Autodesk Inventor part; units mm, degrees
ref_plane "YZ Plane" through (0, 0, 0) normal (1, 0, 0) x (0, 1, 0)
ref_plane "XZ Plane" through (0, 0, 0) normal (0, 1, 0) x (-1, 0, 0)
ref_plane "XY Plane" through (0, 0, 0) normal (0, 0, 1) x (1, 0, 0)
sketch "Sketch1" plane through (0, 0, 0) normal (0, 0, 1) x (1, 0, 0)
  line L0 (-17.5524, 1.6365) -> (20.5476, 1.6365)
  line L1 (20.5476, 1.6365) -> (20.5476, -1.5385)
  line L2 (20.5476, -1.5385) -> (-17.5524, -1.5385)
  line L3 (-17.5524, -1.5385) -> (-17.5524, 1.6365)
  line L4 (-17.5524, -1.5385) -> (-14.3774, -1.5385)
  line L5 (-14.3774, -1.5385) -> (-14.3774, 36.5615)
  line L6 (-14.3774, 36.5615) -> (-17.5524, 36.5615)
  line L7 (-17.5524, 36.5615) -> (-17.5524, -1.5385)
  point P0 (0, 0)
  dimension "d0" = 38.1
  dimension "d1" = 38.1
  dimension "d2" = 3.175
  dimension "d3" = 3.175
extrude "Extrusion1" add sketch "Sketch1" along normal blind 156.21
sketch "Sketch2" plane through (-17.5524, -1.5385, 0) normal (-1, 0, 0) x (0, 0, 1)
  line L0 (156.21, 0) -> (156.21, 38.1)
  line L1 (0, 38.1) -> (0, 0)
  line L2 (0, 0) -> (156.21, 0)
  circle A0 centre (12.7, 7.62) radius 3.175
  circle A1 centre (143.51, 7.62) radius 3.175
  point P0 (0, 1.5385)
  dimension "d6" = 6.35
  dimension "d7" = 6.35
  dimension "d8" = 12.7
  dimension "d9" = 12.7
  dimension "d10" = 7.62
  dimension "d11" = 7.62
extrude "Extrusion2" add sketch "Sketch2" along normal blind 25.4
sketch "Sketch3" plane through (-17.5524, -1.5385, 0) normal (0, -1, 0) x (1, 0, 0)
  line L0 (38.1, 156.21) -> (0, 156.21)
  line L1 (0, 0) -> (0, 156.21)
  line L2 (0, 0) -> (38.1, 0)
  circle A0 centre (7.62, 143.51) radius 3.175
  circle A1 centre (7.62, 12.7) radius 3.175
  point P0 (17.5524, 0)
  dimension "d14" = 12.7
  dimension "d15" = 12.7
  dimension "d16" = 7.62
  dimension "d17" = 7.62
  dimension "d18" = 6.35
  dimension "d19" = 6.35
extrude "Extrusion3" add sketch "Sketch3" along normal blind 25.4
sketch "Sketch4" plane through (-42.9524, 6.0815, 143.51) normal (-1, 0, 0) x (0, 0, 1)
  circle A0 centre (0, 0) radius 3.175
  circle A1 centre (0, 0) radius 9.525
  point P0 (-143.51, -6.0815)
  dimension "d22" = 19.05
extrude "Extrusion4" add sketch "Sketch4" against normal blind 5.5372
sketch "Sketch5" plane through (-42.9524, 6.0815, 12.7) normal (-1, 0, 0) x (0, 0, 1)
  circle A0 centre (0, 0) radius 3.175
  circle A1 centre (0, 0) radius 9.525
  point P0 (-12.7, -6.0815)
  dimension "d25" = 19.05
extrude "Extrusion5" add sketch "Sketch5" against normal blind 5.5372
sketch "Sketch6" plane through (-9.9324, -26.9385, 143.51) normal (0, -1, 0) x (1, 0, 0)
  circle A0 centre (0, 0) radius 3.175
  circle A1 centre (0, 0) radius 9.525
  point P0 (9.9324, -143.51)
  dimension "d28" = 19.05
extrude "Extrusion6" add sketch "Sketch6" against normal blind 5.5372
sketch "Sketch7" plane through (-9.9324, -26.9385, 12.7) normal (0, -1, 0) x (1, 0, 0)
  circle A0 centre (0, 0) radius 3.175
  circle A1 centre (0, 0) radius 9.525
  point P0 (9.9324, -12.7)
  dimension "d31" = 19.05
extrude "Extrusion7" add sketch "Sketch7" against normal blind 5.5372
ref_plane "Work Plane1" through (-17.5524, -1.5385, 0) normal (0.7071, 0.7071, 0) x (0, 0, 1)
sketch "Sketch8" plane through (-17.5524, -1.5385, 0) normal (0.7071, 0.7071, 0) x (0, 0, 1)
  line L0 (156.21, 0) -> (156.21, -26.9408)
  line L1 (0, -26.9408) -> (0, 0)
  line L2 (0, -26.9408) -> (156.21, -26.9408)
  point P0 (0, 11.3236)
  point P1 (38.1, -0.0168)
  point P2 (118.11, -0.0168)
  dimension "d35" = 38.1
  dimension "d36" = 38.1
  dimension "d37" = 26.924
  dimension "d38" = 26.924
equation "\"d7\" = d6"
properties part number "x-bearing assy"
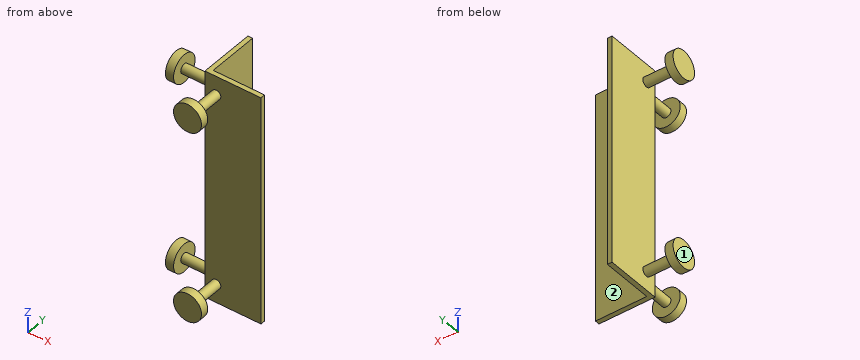
Geometry check sheet. Reference: the model listing, model coordinates, mm. Face numbers are marked on the shaded views. A direction names the side the tool comes from. Coordinates: 2 decimals unless noted, no trailing zeros. Order: outer loops, then holes, each group sorted by start corner. A loop starts at its lowest first (then second) coordinate and runs counter-clockwise, first axis right, second up. Notation, with made-up numbers: (-34.75, -31.5) - (-26.75, -31.5) arc R7 ccw to (-26.75, -26.5) - close; hole circle Ø9 at (47, -14.5). An arc over 180 degrees is marked (long way). Answer in a Markdown table with one row per item. Add a question column.
1. Section check B-B (y = 31). Enter the section's corners in (x, z).
2. Material ranges on L1, parallel to Y at x = -16.5, z = 14; L2, parallel to Y at x = -12.5, z = 142; L3, parallel to Y at x = 10, z = 15, recorded low to high. Write a range as [from, to].
3. Section check D-D (z = 62.5). Enter the section's corners in (x, y), plus the area to 3 significant figures.
4. Gauge pin test, flat ends, axial feed: pin 1 Ø8 at (y, z) = (27, 55) entering from -X; pin 2 Ø17.5 at (x, z) = (10, 75.5) entering from +Y; pin 3 Ø17.5 at (y, z) = (16, 98.5) entering from +X. Record the tip position at first contact, or that the pin passes through.
5. Access from +Z, -Z, +X, -X, +Y, -Y to the whole of each face (thin tool, end or side, straight path). Record for the marked faces 1 and 2.
6. Section check A-A (z = 143.51). Enter the section's corners in (x, y), plus the area to 3 significant figures.
Data:
| question | item | result |
|---|---|---|
| 1 | outline | (-17.55, 0) - (-14.38, 0) - (-14.38, 156.21) - (-17.55, 156.21) - close |
| 2 | L1 | y = [-26.94, -21.4], [-1.54, 36.56] |
| 2 | L2 | y = [-26.94, 1.64] |
| 2 | L3 | y = [-1.54, 1.64] |
| 3 | outline | (-17.55, -1.54) - (20.55, -1.54) - (20.55, 1.64) - (-14.38, 1.64) - (-14.38, 36.56) - (-17.55, 36.56) - close |
| 3 | area | 232 mm² |
| 4 | pin 1 | stops at x = -17.55 |
| 4 | pin 2 | stops at y = 1.64 |
| 4 | pin 3 | stops at x = -14.38 |
| 5 | face 1 | +Z, -Z, -X, +Y, -Y |
| 5 | face 2 | +Z, -Z, +X, +Y |
| 6 | outline | (-42.95, -3.44) - (-37.42, -3.44) - (-37.42, 2.91) - (-17.55, 2.91) - (-17.55, -1.54) - (-13.11, -1.54) - (-13.11, -21.4) - (-19.46, -21.4) - (-19.46, -26.94) - (-0.41, -26.94) - (-0.41, -21.4) - (-6.76, -21.4) - (-6.76, -1.54) - (20.55, -1.54) - (20.55, 1.64) - (-14.38, 1.64) - (-14.38, 36.56) - (-17.55, 36.56) - (-17.55, 9.26) - (-37.42, 9.26) - (-37.42, 15.61) - (-42.95, 15.61) - close |
| 6 | area | 695 mm² |
